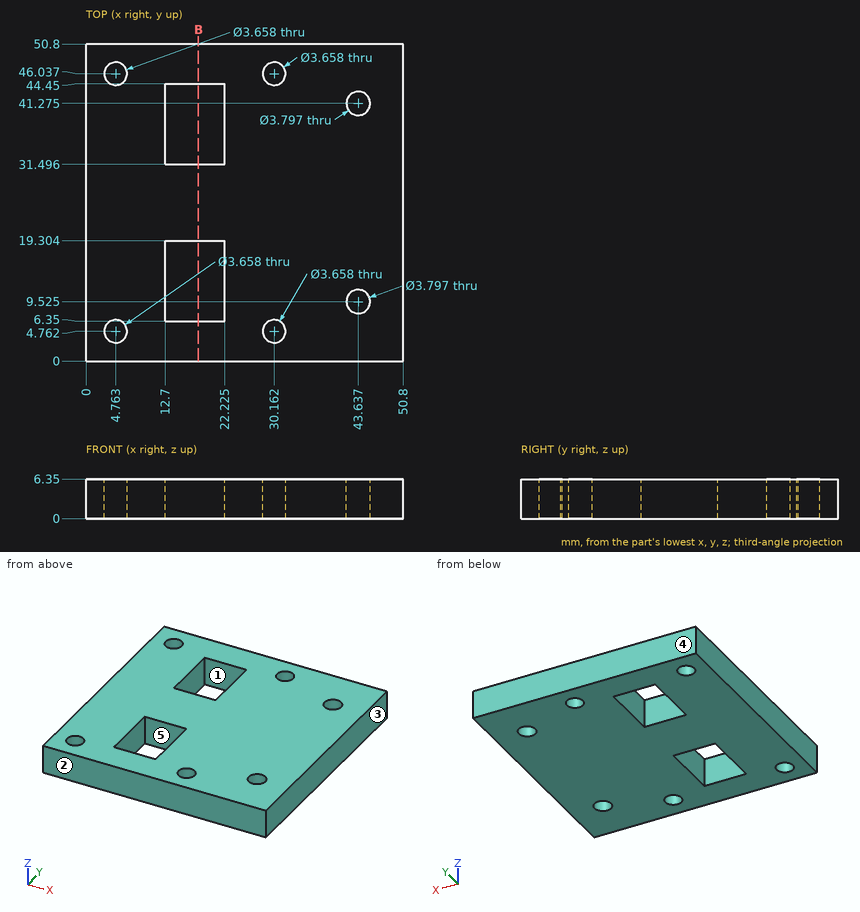
The figure shows three views and two pictorial views of one solid part (mm, origin at its lowest corner). Answer the questions. A direction names the side the tool comes from. Round coordinates to 2 decimals unless told otherwise and drop trailing zeros. Use one line per item in the form item = value. Start each with the question number.
(1) Which of the six approach directions +Z, -Z, +X, -X, +Y, -Y give full straight-line access (tool end or side, diameter ignored) to the marked faces 1 and 2?
(2) Determine the mould class of the marked faces 3, 4 and 5 for opening direction Y: +Y half, -Y half, draft (parallel to the pull), parting line (faces both ways), or undercut.
(3) Find section B-B on x = 18. Give the number of separate pieces and of enclosed holes in the cut face, and give its area (3 significant figures).
(4) Consider line 1 (Y direction, x = 43.5, z = 1); line 2 (X direction, y = 14.5, z = 2.5) (1 decimal); line 3 (Y direction, x = 31.5, z = 1) (1 decimal). Determine where each line is inside the solid, lowest interval first.
Answer list:
q1.face_1 = +Z, -Z
q1.face_2 = +Z, -Z, +X, -X, -Y
q2.face_3 = draft
q2.face_4 = +Y half
q2.face_5 = undercut
q3.separate_pieces = 3
q3.enclosed_holes = 0
q3.area = 158 mm^2
q4.line_1 = 0 to 7.63, 11.42 to 39.38, 43.17 to 50.8
q4.line_2 = 0 to 12.7, 22.2 to 50.8
q4.line_3 = 0 to 3.5, 6 to 44.8, 47.3 to 50.8
